Build history of the part. All positions in model axes, mm. A direction names the side the tool comes from. Round coordinates to 2 decimals unless told otherwise and drop trailing zeros. Loops run counter-clockwise (first coordinate to the right, second up) from the corner with the lowest first, then second, coordinate; pieces in that order, holes last. Notation, with made-up numbers: (77.25, 49) - (136.25, 49) arc R32 cw to (136.25, 87) - close; hole circle Ø7 at (42, 19). An arc over 180 degrees is marked (long way). Use a Markdown table: item, result.
from build123d import *

# Parameters (mm, degrees)
F0_R     = 0.75
F0_R_2   = 1.45
F1_DEPTH = 2.62
F2_R     = 4.4
F2_R_2   = 2.5
F3_DEPTH = 3
F4_DEPTH = 0.17


with BuildPart() as f1:
    # F0 (on Top) → F1 (new body)
    with BuildSketch(Plane.XY):
        with BuildLine():
            Line((3.95, -3.95), (7.7637545764, -3.95))
            Line((7.7637545764, -3.95), (16.8139215854, -2.0355203167))
            ThreePointArc((16.8139215854, -2.0355203167), (17.9536800138, -1.3382178935), (18.4, -0.0788218419))
            Line((18.4, -0.0788218419), (18.4, 0.0788218419))
            ThreePointArc((18.4, 0.0788218419), (17.9536800138, 1.3382178935), (16.8139215854, 2.0355203167))
            Line((16.8139215854, 2.0355203167), (7.7637545764, 3.95))
            Line((7.7637545764, 3.95), (3.95, 3.95))
            Line((3.95, 3.95), (3.95, 7.6887742616))
            Line((3.95, 7.6887742616), (2.033754464, 16.8111469309))
            ThreePointArc((2.033754464, 16.8111469309), (1.3369682429, 17.9527868273), (0.0764710913, 18.4))
            Line((0.0764710913, 18.4), (-0.0814896041, 18.4))
            ThreePointArc((-0.0814896041, 18.4), (-1.3396337634, 17.9546939488), (-2.0375187153, 16.8170732745))
            Line((-2.0375187153, 16.8170732745), (-3.95, 7.8477403149))
            Line((-3.95, 7.8477403149), (-3.95, 3.95))
            Line((-3.95, 3.95), (-7.7637545764, 3.95))
            Line((-7.7637545764, 3.95), (-16.8139215854, 2.0355203167))
            ThreePointArc((-16.8139215854, 2.0355203167), (-17.9536800138, 1.3382178935), (-18.4, 0.0788218419))
            Line((-18.4, 0.0788218419), (-18.4, -0.0788218419))
            ThreePointArc((-18.4, -0.0788218419), (-17.9536800138, -1.3382178935), (-16.8139215854, -2.0355203167))
            Line((-16.8139215854, -2.0355203167), (-7.7637545764, -3.95))
            Line((-7.7637545764, -3.95), (-3.95, -3.95))
            Line((-3.95, -3.95), (-3.95, -7.8477403149))
            Line((-3.95, -7.8477403149), (-2.0375187153, -16.8170732745))
            ThreePointArc((-2.0375187153, -16.8170732745), (-1.3396337634, -17.9546939488), (-0.0814896041, -18.4))
            Line((-0.0814896041, -18.4), (0.0764710913, -18.4))
            ThreePointArc((0.0764710913, -18.4), (1.3369682429, -17.9527868273), (2.033754464, -16.8111469309))
            Line((2.033754464, -16.8111469309), (3.95, -7.6887742616))
            Line((3.95, -7.6887742616), (3.95, -3.95))
        make_face()
        with Locations((0, -16.4)):
            Circle(F0_R, mode=Mode.SUBTRACT)
        with Locations((0, -13.4)):
            Circle(F0_R, mode=Mode.SUBTRACT)
        with Locations((0, -10.4)):
            Circle(F0_R, mode=Mode.SUBTRACT)
        with Locations((0, -7.4)):
            Circle(F0_R, mode=Mode.SUBTRACT)
        with Locations((-16.4, 0)):
            Circle(F0_R, mode=Mode.SUBTRACT)
        with Locations((-13.4, 0)):
            Circle(F0_R, mode=Mode.SUBTRACT)
        with Locations((-10.4, 0)):
            Circle(F0_R, mode=Mode.SUBTRACT)
        with Locations((-7.4, 0)):
            Circle(F0_R, mode=Mode.SUBTRACT)
        Circle(F0_R_2, mode=Mode.SUBTRACT)
        with Locations((7.4, 0)):
            Circle(F0_R, mode=Mode.SUBTRACT)
        with Locations((0, 7.4)):
            Circle(F0_R, mode=Mode.SUBTRACT)
        with Locations((10.4, 0)):
            Circle(F0_R, mode=Mode.SUBTRACT)
        with Locations((13.4, 0)):
            Circle(F0_R, mode=Mode.SUBTRACT)
        with Locations((16.4, 0)):
            Circle(F0_R, mode=Mode.SUBTRACT)
        with Locations((0, 10.4)):
            Circle(F0_R, mode=Mode.SUBTRACT)
        with Locations((0, 13.4)):
            Circle(F0_R, mode=Mode.SUBTRACT)
        with Locations((0, 16.4)):
            Circle(F0_R, mode=Mode.SUBTRACT)
    extrude(amount=F1_DEPTH)

    # F2 (on face) → F3 (join)
    with BuildSketch(Plane(origin=(0, 0, 0), x_dir=(1, 0, 0), z_dir=(0, 0, -1))):
        Circle(F2_R)
        Circle(F2_R_2, mode=Mode.SUBTRACT)
    extrude(amount=F3_DEPTH)

    # F4 (cut): a face of the model
    f4_faces = [f1.faces().sort_by_distance(p)[0] for p in [
        (-2.4292893219, 0, 0),
    ]]
    extrude(f4_faces, amount=-F4_DEPTH, mode=Mode.SUBTRACT)


solid = f1.part
Q1. Which spindle directions (+Z, -Z, +X, -X, +Y, -Y) get a long thin tool onto all of the face, cutting with end or side? Do faces 1 (the face through (-3.95, 6, 1)), 2 (the face through (-0.54, 2.44, -1.39)), 3 (the face through (-6, -3.95, 1)), 4 (the face through (3.95, -6, 1)). Say none if no direction does.
Results found:
| item | result |
|---|---|
| face 1 | +Z, -Z, -X, +Y |
| face 2 | -Z |
| face 3 | +Z, -Z, -X, -Y |
| face 4 | +Z, -Z, +X, -Y |
Q2. Probe line 1 (Y direction, x = -7.4, z = 1.9); line 2 (X direction, y = 7.5, z = 0.15); line 3 (Z direction, x = 1, y = 16). List the from-to ranges inside material, lowest first.
Results found:
| item | result |
|---|---|
| line 1 | y = -3.95 to -0.75, 0.75 to 3.95 |
| line 2 | x = -3.95 to -0.74, 0.74 to 3.95 |
| line 3 | z = 0 to 2.62 |
Q3. Drop flat-ended pins along their axis: pin 1 (2 mm diameter, centred on x = 5.5, z = 1.5, fed in from +Y); pin 2 (2 mm diameter, centred on x = -7.4, y = 0, fed in from -Z); pin 3 (0.8 mm diameter, centred on y = -6.5, z = 2, fed in from -X). Give the stop position or say it passes through.
Results found:
| item | result |
|---|---|
| pin 1 | stops at y = 3.95 |
| pin 2 | stops at z = 0 |
| pin 3 | stops at x = -3.95 |
Q4. Pull direction X, two halves, no side cores. Call faces 5 (the face through (-17.9, 1.4, 1.3)), 6 (the face through (-12.685, 0.225, 1.292)), 7 (the face through (2, 2, -3)), 8 (the face through (12.35, 2.98, 1.29)): pulls with the +X half, pulls with the -X half, needs draft (parallel to the pull), parting line crosses it, or undercut.
Results found:
| item | result |
|---|---|
| face 5 | pulls with the -X half |
| face 6 | undercut |
| face 7 | needs draft |
| face 8 | pulls with the +X half |
Q5. Cut at A-A, the plane x = -10.4. List the corners of the cut face in (y, z), plus the area to 3 significant figures.
Results found:
| item | result |
|---|---|
| outline | (-3.39, 0) - (-0.75, 0) - (-0.75, 2.62) - (-3.39, 2.62) - close; (0.75, 0) - (3.39, 0) - (3.39, 2.62) - (0.75, 2.62) - close |
| area | 13.8 mm2 |
Q6. Cut at C-C, the plane y = -3. List the corners of the cut face in (x, z).
Results found:
| item | result |
|---|---|
| outline | (-12.25, 0) - (-3.22, 0) - (-3.22, -3) - (3.22, -3) - (3.22, 0) - (12.25, 0) - (12.25, 2.62) - (-12.25, 2.62) - close |
Q7. Cut at B-B, the plane y = 13.4. List the corners of the cut face in (x, z).
Results found:
| item | result |
|---|---|
| outline | (-2.77, 0) - (-0.75, 0) - (-0.75, 2.62) - (-2.77, 2.62) - close; (0.75, 0) - (2.75, 0) - (2.75, 2.62) - (0.75, 2.62) - close |
Q8. Cut at D-D, the plane y = 6. List the corners of the cut face in (x, z), plus the area to 3 significant figures.
Results found:
| item | result |
|---|---|
| outline | (-3.95, 0) - (3.95, 0) - (3.95, 2.62) - (-3.95, 2.62) - close |
| area | 20.7 mm2 |
